Check sheet for the modelled part. Datum: model origin and axes. Units: mm. A direction names the side the tool comes from. Coordinates: 2 decimals unless noted, no trailing zeros. Loops run counter-clockwise (first coordinate to the right, second up) from the corner with the lowest first, then second, coordinate; pieces in that order, holes last. Notation, with made-up numbers: (-3.75, 36.5) -> (45.25, 36.5) arc R17 ccw to (45.25, 42.5) -> close; hole circle Ø2 at (72, 45.5). An arc over 180 degrees is marked (long way). Use CSV: the item, a comma, the result in double quotes. Start each with the question number.
1. Sectioned sample at A-A, the plane y = 37.5. Count the separate pieces of the cut face and the enclosed holes in it, and give its area (3 significant figures).
2. Gauge pin test, flat ends, axial feed: pin 1 (6 mm diameter, centred on x = 50, z = 8, fed in from -Y); pin 2 (1.5 mm diameter, centred on y = 25, z = 20, fed in from +X); pin 3 (8 mm diameter, centred on y = 22.5, z = 20, fed in from -X). Record the tip position at first contact, or that the pin passes through.
3. Release check for a two-part mould opening along X. For faces 4 (the face through (91, 26.5, 20)), 5 (the face through (-2, 50, 20)), 6 (the face through (-43, 13, 20)), 7 (the face through (-147, 25, 7)) record: pulls with the +X half, pulls with the -X half, needs draft (parallel to the pull), parting line crosses it, or undercut.
4. Set-up check for faces 1 (the face through (-49, 26.5, 20)), 2 (the face through (122, 0, 11)), 3 (the face through (-128.486, 15.703, 32.395)): record each of +Z, -Z, +X, -X, +Y, -Y from which the full face is reachable in a straight line by a thin tool's end or side.
5. Sectioned sample at B-B, the plane x = 90. Record the cut outline in (y, z).
6. Thickness scan on L1, parallel to X at y = 22, z = 18.5; L2, parallel to Y at x = -114.5, z = 7; L3, parallel to X at y = 44, z = 8. Record the ranges inside material, lowest first.
7. Sectioned sample at C-C, the plane x = -137. Record the cut outline in (y, z).
```python
from build123d import *

# Parameters (mm, degrees)
SKETCH1_R           = 2.5
BOSS_EXTRUDE1_DEPTH = 40
SKETCH3_R           = 2.5
CUT_EXTRUDE2_DEPTH  = 23.5
CUT_EXTRUDE3_REACH  = 162.34
SKETCH4_W           = 40
SKETCH4_H           = 10


with BuildPart() as part:
    # Sketch1 → Boss-Extrude1 (new body)
    with BuildSketch(Plane.XY):
        with BuildLine():
            Line((0, 50), (0, 0))
            Line((0, 0), (43, 0))
            Line((43, 0), (43, 26.5))
            Line((43, 26.5), (55.075188443, 26.5))
            ThreePointArc((55.075188443, 26.5), (70, 40), (84.924811557, 26.5))
            Line((84.924811557, 26.5), (97, 26.5))
            Line((97, 26.5), (97, 0))
            Line((97, 0), (147, 0))
            Line((147, 0), (147, 50))
            Line((147, 50), (62, 50))
            Line((62, 50), (23, 50))
            Line((23, 50), (0, 50))
        make_face()
        with BuildLine():
            ThreePointArc((139.5, 30), (132.17766953, 12.32233047), (114.5, 5))
            ThreePointArc((114.5, 5), (112, 7.5), (114.5, 10))
            ThreePointArc((114.5, 10), (128.642135624, 15.857864376), (134.5, 30))
            ThreePointArc((134.5, 30), (137, 32.5), (139.5, 30))
        make_face(mode=Mode.SUBTRACT)
        with Locations((114.5, 30)):
            Circle(SKETCH1_R, mode=Mode.SUBTRACT)
    boss_extrude1 = extrude(amount=BOSS_EXTRUDE1_DEPTH)

    # Sketch3 → Cut-Extrude2 (cut)
    with BuildSketch(Plane(origin=(0, 50, 0), x_dir=(1, 0, 0), z_dir=(0, 1, 0))):
        with Locations(Location((50, -32, 0), (0, 0, 270))):
            Circle(SKETCH3_R)
        with Locations(Location((90, -32, 0), (0, 0, 270))):
            Circle(SKETCH3_R)
        with Locations(Location((50, -8, 0), (0, 0, 270))):
            Circle(SKETCH3_R)
        with Locations(Location((90, -8, 0), (0, 0, 270))):
            Circle(SKETCH3_R)
    cut_extrude2 = extrude(amount=-CUT_EXTRUDE2_DEPTH, mode=Mode.SUBTRACT)

    # Cut-Extrude3: up to this face of the body (flat: up to its plane)
    cut_extrude3_end = Plane(part.part.faces().sort_by_distance((122, 0, 20))[0])
    # Sketch4 → Cut-Extrude3 (cut, up to the picked face)
    with BuildSketch(Plane(origin=(0, 50, 0), x_dir=(1, 0, 0), z_dir=(0, 1, 0)), mode=Mode.PRIVATE) as cut_extrude3_sk1:
        with Locations((127, -20)):
            Rectangle(SKETCH4_W, SKETCH4_H)
    cut_extrude3_tool1 = split(extrude(cut_extrude3_sk1.sketch, amount=-CUT_EXTRUDE3_REACH, mode=Mode.PRIVATE), bisect_by=cut_extrude3_end, keep=Keep.BOTH, mode=Mode.PRIVATE)
    cut_extrude3 = cut_extrude3_tool1.solids().sort_by(Axis((127, 50, 20), (0, -1, 0)))[0]
    add(cut_extrude3, mode=Mode.SUBTRACT)

    # Mirror2: Boss-Extrude1, Cut-Extrude2, Cut-Extrude3 across plane
    add(boss_extrude1.mirror(Plane(origin=(0, 0, 40), x_dir=(0, 0, 1), z_dir=(-1, 0, 0))))
    add(cut_extrude2.mirror(Plane(origin=(0, 0, 40), x_dir=(0, 0, 1), z_dir=(-1, 0, 0))), mode=Mode.SUBTRACT)
    add(cut_extrude3.mirror(Plane(origin=(0, 0, 40), x_dir=(0, 0, 1), z_dir=(-1, 0, 0))), mode=Mode.SUBTRACT)


solid = part.part
```
Completed:
1,separate pieces,"3"
1,enclosed holes,"8"
1,area,"9,480 mm²"
2,pin 1,"y = 26.5"
2,pin 2,"x = 107"
2,pin 3,"x = -107"
3,face 4,"undercut"
3,face 5,"needs draft"
3,face 6,"undercut"
3,face 7,"pulls with the -X half"
4,face 1,"+Z, -Z, -Y"
4,face 2,"+Z, -Z, +X, -X, -Y"
4,face 3,"+Z, -Z"
5,outline,"(26.5, 0) -> (50, 0) -> (50, 5.5) -> (26.5, 5.5) -> close; (26.5, 10.5) -> (50, 10.5) -> (50, 29.5) -> (26.5, 29.5) -> close; (26.5, 34.5) -> (50, 34.5) -> (50, 40) -> (26.5, 40) -> close"
6,L1,"-107 to -97, -43 to 43, 97 to 107"
6,L2,"0 to 5, 10 to 27.5, 32.5 to 50"
6,L3,"-147 to -92.5, -87.5 to -52.5, -47.5 to 47.5, 52.5 to 87.5, 92.5 to 147"
7,outline,"(0, 0) -> (19.1, 0) -> (19.1, 15) -> (0, 15) -> close; (0, 25) -> (19.1, 25) -> (19.1, 40) -> (0, 40) -> close; (32.5, 0) -> (50, 0) -> (50, 15) -> (32.5, 15) -> close; (32.5, 25) -> (50, 25) -> (50, 40) -> (32.5, 40) -> close"
